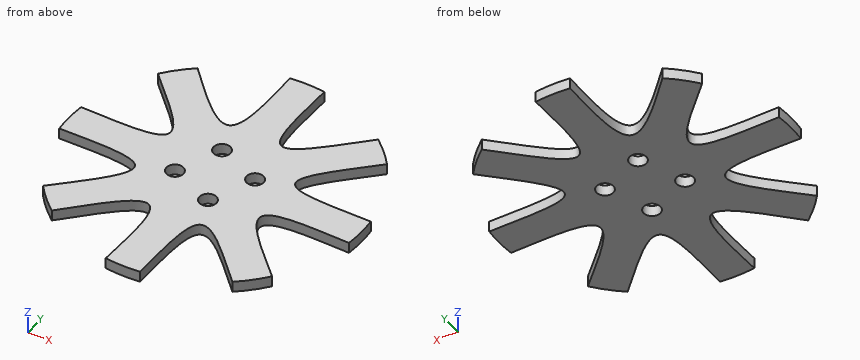
from build123d import *

# Parameters (mm, degrees)
F0_R     = 1.2446
F1_DEPTH = 0.79375
F6_DEPTH = 1.5875


with BuildPart() as f1:
    # F0 (on Top) → F1 (new body, symmetric)
    with BuildSketch(Plane.XY):
        with BuildLine():
            ThreePointArc((-13.3643659864, 16.9564684348), (-15.2664354058, 15.2664354058), (-16.9564684348, 13.3643659864))
            ThreePointArc((-16.9564684348, 13.3643659864), (-16.6604544533, 6.9009861898), (-21.4400676305, 2.54))
            ThreePointArc((-21.4400676305, 2.54), (-21.59, 0), (-21.4400676305, -2.54))
            ThreePointArc((-21.4400676305, -2.54), (-16.6604544533, -6.9009861898), (-16.9564684348, -13.3643659864))
            ThreePointArc((-16.9564684348, -13.3643659864), (-15.2664354058, -15.2664354058), (-13.3643659864, -16.9564684348))
            ThreePointArc((-13.3643659864, -16.9564684348), (-6.9009861898, -16.6604544533), (-2.54, -21.4400676305))
            ThreePointArc((-2.54, -21.4400676305), (0, -21.59), (2.54, -21.4400676305))
            ThreePointArc((2.54, -21.4400676305), (6.9009861898, -16.6604544533), (13.3643659864, -16.9564684348))
            ThreePointArc((13.3643659864, -16.9564684348), (15.2664354058, -15.2664354058), (16.9564684348, -13.3643659864))
            ThreePointArc((16.9564684348, -13.3643659864), (16.6604544533, -6.9009861898), (21.4400676305, -2.54))
            ThreePointArc((21.4400676305, -2.54), (21.59, 0), (21.4400676305, 2.54))
            ThreePointArc((21.4400676305, 2.54), (16.6604544533, 6.9009861898), (16.9564684348, 13.3643659864))
            ThreePointArc((16.9564684348, 13.3643659864), (15.2664354058, 15.2664354058), (13.3643659864, 16.9564684348))
            ThreePointArc((13.3643659864, 16.9564684348), (6.9009861898, 16.6604544533), (2.54, 21.4400676305))
            ThreePointArc((2.54, 21.4400676305), (0, 21.59), (-2.54, 21.4400676305))
            ThreePointArc((-2.54, 21.4400676305), (-6.9009861898, 16.6604544533), (-13.3643659864, 16.9564684348))
        make_face()
        with Locations((-4.6933080252, -1.9440318364)):
            Circle(F0_R, mode=Mode.SUBTRACT)
        with Locations((1.9440318364, -4.6933080252)):
            Circle(F0_R, mode=Mode.SUBTRACT)
        with Locations((-1.9440318364, 4.6933080252)):
            Circle(F0_R, mode=Mode.SUBTRACT)
        with Locations((4.6933080252, 1.9440318364)):
            Circle(F0_R, mode=Mode.SUBTRACT)
    extrude(amount=F1_DEPTH, both=True)

    # F5 (on face) → F6 (cut, through all)
    with BuildSketch(Plane.XY.offset(0.79375)):
        with BuildLine():
            ThreePointArc((21.4400676305, 2.54), (16.6604544533, 6.9009861898), (16.9564684348, 13.3643659864))
            add(Edge.make_bspline(
                [(16.9564684348, 13.3643659864), (12.7702234313, 9.1661904007), (4.5537464117, 1.9143787537), (15.6687479466, 2.5573067833), (21.4400676305, 2.54)],
                knots=[0, 0, 0, 0, 0.5, 1, 1, 1, 1], degree=3))
        make_face()
        with BuildLine():
            ThreePointArc((2.54, -21.4400676305), (6.9009861898, -16.6604544533), (13.3643659864, -16.9564684348))
            add(Edge.make_bspline(
                [(2.54, -21.4400676305), (2.5372293312, -15.7558191568), (1.8345788445, -4.4215889444), (9.3458676711, -12.9474671558), (13.3643659864, -16.9564684348)],
                knots=[0, 0, 0, 0, 0.5, 1, 1, 1, 1], degree=3))
        make_face()
        with BuildLine():
            ThreePointArc((16.9564684348, -13.3643659864), (16.6604544533, -6.9009861898), (21.4400676305, -2.54))
            add(Edge.make_bspline(
                [(21.4400676305, -2.54), (16.1842592061, -2.4963843171), (4.082315581, -1.6922755491), (13.1975738332, -9.6713192761), (16.9564684348, -13.3643659864)],
                knots=[0, 0, 0, 0, 0.5, 1, 1, 1, 1], degree=3))
        make_face()
        with BuildLine():
            ThreePointArc((-13.3643659864, -16.9564684348), (-6.9009861898, -16.6604544533), (-2.54, -21.4400676305))
            add(Edge.make_bspline(
                [(-13.3643659864, -16.9564684348), (-9.9083529785, -13.3942691609), (-1.5885540375, -3.8302056287), (-2.4667936377, -16.4917837828), (-2.54, -21.4400676305)],
                knots=[0, 0, 0, 0, 0.5, 1, 1, 1, 1], degree=3))
        make_face()
        with BuildLine():
            add(Edge.make_bspline(
                [(2.54, 21.4400676305), (2.5480384938, 15.6409479678), (1.8768956976, 4.5266398025), (9.2504248023, 12.8522366285), (13.3643659864, 16.9564684348)],
                knots=[0, 0, 0, 0, 0.5, 1, 1, 1, 1], degree=3))
            ThreePointArc((13.3643659864, 16.9564684348), (6.9009861898, 16.6604544533), (2.54, 21.4400676305))
        make_face()
        with BuildLine():
            add(Edge.make_bspline(
                [(-13.3643659864, 16.9564684348), (-10.1164951921, 13.5911004618), (-1.4928890483, 3.6003961955), (-2.4499814026, 16.7545713484), (-2.54, 21.4400676305)],
                knots=[0, 0, 0, 0, 0.5, 1, 1, 1, 1], degree=3))
            ThreePointArc((-2.54, 21.4400676305), (-6.9009861898, 16.6604544533), (-13.3643659864, 16.9564684348))
        make_face()
        with BuildLine():
            add(Edge.make_bspline(
                [(-16.9564684348, 13.3643659864), (-12.9633266479, 9.4111068174), (-4.3837218341, 1.8060450999), (-15.8156938851, 2.5290576741), (-21.4400676305, 2.54)],
                knots=[0, 0, 0, 0, 0.5, 1, 1, 1, 1], degree=3))
            ThreePointArc((-16.9564684348, 13.3643659864), (-16.6604544533, 6.9009861898), (-21.4400676305, 2.54))
        make_face()
        with BuildLine():
            add(Edge.make_bspline(
                [(-21.4400676305, -2.54), (-16.1078236997, -2.4722644594), (-4.1337008384, -1.7207956731), (-13.1712388247, -9.6383988857), (-16.9564684348, -13.3643659864)],
                knots=[0, 0, 0, 0, 0.5, 1, 1, 1, 1], degree=3))
            ThreePointArc((-21.4400676305, -2.54), (-16.6604544533, -6.9009861898), (-16.9564684348, -13.3643659864))
        make_face()
    extrude(amount=-F6_DEPTH, mode=Mode.SUBTRACT)


solid = f1.part
Geometry: final body of the model. Coordinates: model frame, mm. Give positions to 0.01 mm unless a question says otherwise; leave off trailing zeros. Loops run counter-clockwise (first coordinate to the right, second up) from the corner with the lowest first, then second, coordinate; pieces in that order, holes last. Notation, with made-up numbers: (80.5, 1) - (95.5, 1) arc R10 cw to (95.5, 16) - close; hole circle Ø2 at (6.25, 70). An arc over 180 degrees is marked (long way). Answer as CSV lines item,"result". Start each with the question number.
1. Pin query (flat end, axial travel): P1, Ø4, axis at x = 4.69, y = 1.94, coming from the -Z side; P2, Ø1, axis at x = -12.5, y = -6.5, coming from the -Z side. Return the tip coordinate at first contact, or that it passes through.
2. Ray query, L1, parallel to X at y = 13, z = -0.1; L2, parallel to Y at x = 10, z = -0.35; L3, parallel to Y at x = -11, z = 0.35. Return the intervals inside material, ascending.
3. Section A-A, the plane x = 1.5. Return loops of the section in (y, z).
4. Section B-B, the plane x = -12.5. Give the number of separate pieces and of enclosed holes in the cut face, plus the area to 3 significant figures.
Answers:
1,P1,"stops at z = -0.79"
1,P2,"passes through"
2,L1,"x = -16.59 to -9.57, -2.52 to 2.62, 9.44 to 16.59"
2,L2,"y = -13.55 to -6.06, -3.25 to 3.28, 6.01 to 13.56"
2,L3,"y = -14.49 to -7.36, -2.87 to 2.89, 7.32 to 14.47"
3,outline,"(-21.54, -0.79) - (-5.86, -0.79) - (-5.86, 0.79) - (-21.54, 0.79) - close; (-3.53, -0.79) - (21.54, -0.79) - (21.54, 0.79) - (-3.53, 0.79) - close"
4,separate pieces,"3"
4,enclosed holes,"0"
4,area,"30.8 mm2"
